Check sheet for the modelled part. Datum: model origin and axes. Units: mm. A direction names the side the tool comes from. Give positions to 0.01 mm unless a question says otherwise; leave off trailing zeros. Write each loop counter-clockwise with the first axis right and the second up, starting at its lowest first coordinate (ties: lowest second). Pieces come first, ordered by that corner, then holes. Notation, with made-up numbers: (-29, -30) -> (-12, -30) arc R37 ccw to (-12, 7) -> close; hole circle Ø5 at (45.25, 1). An arc over 180 degrees is marked (long way). Answer as a JSON object with one key per item and string values.
from build123d import *

# Parameters (mm, degrees)
SKETCH2_R           = 1.249995
BOSS_EXTRUDE1_DEPTH = 1.5875


with BuildPart() as part:
    # Sketch2 → Boss-Extrude1 (new body)
    with BuildSketch(Plane.XY):
        with BuildLine():
            Line((64.000000001, -40.999999999), (64.000000001, 37.999999999))
            Line((64.000000001, 37.999999999), (59.000000001, 42.999999999))
            Line((59.000000001, 42.999999999), (-62, 42.999999999))
            ThreePointArc((-62, 42.999999999), (-63.414213563, 42.414213561), (-64.000000001, 40.999999999))
            Line((-64.000000001, 40.999999999), (-64.000000001, 35.5))
            Line((-64.000000001, 35.5), (-54.500000001, 35.5))
            Line((-54.500000001, 35.5), (-54.500000001, 29.086543683))
            Line((-54.500000001, 29.086543683), (-9.009111538, 0.298612306))
            Line((-9.009111538, 0.298612306), (-54.500000001, -28.57300784))
            Line((-54.500000001, -28.57300784), (-54.500000001, -35.5))
            Line((-54.500000001, -35.5), (-64.000000001, -35.5))
            Line((-64.000000001, -35.5), (-64.000000001, -40.999999999))
            ThreePointArc((-64.000000001, -40.999999999), (-63.414213563, -42.414213561), (-62, -42.999999999))
            Line((-62, -42.999999999), (62, -42.999999999))
            ThreePointArc((62, -42.999999999), (63.414213563, -42.414213561), (64.000000001, -40.999999999))
        make_face()
        with Locations((59.000000001, -38)):
            Circle(SKETCH2_R, mode=Mode.SUBTRACT)
        with Locations((-59.000000001, -38)):
            Circle(SKETCH2_R, mode=Mode.SUBTRACT)
        with Locations((59.000000001, 37.999999999)):
            Circle(SKETCH2_R, mode=Mode.SUBTRACT)
        with Locations((-59.000000001, 37.999999999)):
            Circle(SKETCH2_R, mode=Mode.SUBTRACT)
        Polygon((-45.624235778, 34.999999999), (45.667312892, 34.999999999), (0.200195404, 6.143466535), align=None, mode=Mode.SUBTRACT)
        Polygon((-45.681229003, -34.999999999), (46.769999999, -34.999999999), (0.409618796, -5.661828822), align=None, mode=Mode.SUBTRACT)
        Polygon((55.000000001, 29.086543683), (55.000000001, -28.365033721), (9.628517212, 0.206269351), align=None, mode=Mode.SUBTRACT)
    extrude(amount=BOSS_EXTRUDE1_DEPTH)


solid = part.part
1. Sectioned sample at A-A, the plane y = -38. Enter the section's corners in (x, z), plus the area to 3 significant figures.
Determined:
{"outline": "(-64, 0) -> (-60.25, 0) -> (-60.25, 1.59) -> (-64, 1.59) -> close; (-57.75, 0) -> (57.75, 0) -> (57.75, 1.59) -> (-57.75, 1.59) -> close; (60.25, 0) -> (64, 0) -> (64, 1.59) -> (60.25, 1.59) -> close", "area": "195 mm^2"}
2. Sectioned sample at C-C, the plane z = 1. Enter the section's corners in (x, y).
Determined:
{"outline": "(-64, -41) arc R2 ccw to (-62, -43) -> (62, -43) arc R2 ccw to (64, -41) -> (64, 38) -> (59, 43) -> (-62, 43) arc R2 ccw to (-64, 41) -> (-64, 35.5) -> (-54.5, 35.5) -> (-54.5, 29.09) -> (-9.01, 0.3) -> (-54.5, -28.57) -> (-54.5, -35.5) -> (-64, -35.5) -> close; hole circle Ø2.5 at (-59, -38); hole circle Ø2.5 at (-59, 38); hole (-45.68, -35) -> (46.77, -35) -> (0.41, -5.66) -> close; hole (-45.62, 35) -> (0.2, 6.14) -> (45.67, 35) -> close; hole (9.63, 0.21) -> (55, -28.37) -> (55, 29.09) -> close; hole circle Ø2.5 at (59, -38); hole circle Ø2.5 at (59, 38)"}
3. Sectioned sample at B-B, the plane x = -59. Enter the section's corners in (y, z), plus the area to 3 significant figures.
Determined:
{"outline": "(-43, 0) -> (-39.25, 0) -> (-39.25, 1.59) -> (-43, 1.59) -> close; (-36.75, 0) -> (-35.5, 0) -> (-35.5, 1.59) -> (-36.75, 1.59) -> close; (35.5, 0) -> (36.75, 0) -> (36.75, 1.59) -> (35.5, 1.59) -> close; (39.25, 0) -> (43, 0) -> (43, 1.59) -> (39.25, 1.59) -> close", "area": "15.9 mm^2"}
4. Sectioned sample at D-D, the plane y = 3. Enter the section's corners in (x, z), plus the area to 3 significant figures.
Determined:
{"outline": "(-13.28, 0) -> (14.02, 0) -> (14.02, 1.59) -> (-13.28, 1.59) -> close; (55, 0) -> (64, 0) -> (64, 1.59) -> (55, 1.59) -> close", "area": "57.6 mm^2"}
5. Scan lines: L1, parallel to X at y = 38, z = 0.75; L2, parallel to Y at x = -59, z = 0.4; L3, parallel to Y at x = -10.5, z = 1. Record each from-to range of solid material in increasing order. Write a range as [from, to].
Determined:
{"L1": "[-64, -60.25], [-57.75, 57.75], [60.25, 64]", "L2": "[-43, -39.25], [-36.75, -35.5], [35.5, 36.75], [39.25, 43]", "L3": "[-43, -35], [-12.61, -0.65], [1.24, 12.88], [35, 43]"}
6. Access from +Z, -Z, +X, -X, +Y, -Y to the whole of each face (thin tool, end or side, straight path). Record for faces 5 (the face through (32.63, -14.28, 0.78)), 6 (the face through (13, 10, 0)), 7 (the face through (-31.436, -13.935, 0.783)).
Determined:
{"face 5": "+Z, -Z", "face 6": "-Z, +X, -X, +Y, -Y", "face 7": "+Z, -Z, -X"}
7. Mould release check, pull along X, two halves, no side actions. Record for faces 1 (the face through (-59.99, 37.24, 0.78)), 2 (the face through (62, 40, 1)), 3 (the face through (13, 10, 1.588)), 4 (the face through (-22.313, -20.126, 0.783)): released by +X, released by -X, zero draft, split by the parting line, or undercut.
Determined:
{"face 1": "undercut", "face 2": "released by +X", "face 3": "zero draft", "face 4": "undercut"}
